Work out the finished part from the listing and answer in its coordinate system (mm). A direction names the side the tool comes from. Give positions to 0.01 mm unless a question says otherwise; leave off trailing zeros. Order: outer loops, then holes, each group sorted by start corner. A loop starts at its lowest first (then second) coordinate and runs counter-clockwise, first axis right, second up.
```python
from build123d import *

# Parameters (mm, degrees)
CROQUIS1_R              = 4
CROQUIS1_R_2            = 3
SALIENTE_EXTRUIR1_DEPTH = 5.5
CROQUIS2_R              = 5.35
CROQUIS2_R_2            = 3
SALIENTE_EXTRUIR2_DEPTH = 2.5
REDONDEO1_R             = 1
CROQUIS3_R              = 4
SALIENTE_EXTRUIR3_DEPTH = 7
CROQUIS4_W              = 2.8
CROQUIS4_H              = 0.7
CROQUIS4_W_2            = 0.7
CROQUIS4_H_2            = 2.8
SALIENTE_EXTRUIR4_DEPTH = 5.3
CROQUIS5_R              = 4
SALIENTE_EXTRUIR5_DEPTH = 2


with BuildPart() as part:
    # Croquis1 → Saliente-Extruir1 (new body)
    with BuildSketch(Plane.XY):
        Circle(CROQUIS1_R)
        Circle(CROQUIS1_R_2, mode=Mode.SUBTRACT)
    extrude(amount=-SALIENTE_EXTRUIR1_DEPTH)

    # Croquis2 → Saliente-Extruir2 (add)
    with BuildSketch(Plane(origin=(0, 0, -5.5), x_dir=(-1, 0, 0), z_dir=(0, 0, -1))):
        Circle(CROQUIS2_R)
        with Locations(Location((0, 0, 0), (0, 0, 180))):
            Circle(CROQUIS2_R_2, mode=Mode.SUBTRACT)
    extrude(amount=SALIENTE_EXTRUIR2_DEPTH)

    # Redondeo1
    redondeo1_edges = [part.edges().sort_by_distance(p)[0] for p in [
        (5.35, 0, -8),
    ]]
    fillet(redondeo1_edges, radius=REDONDEO1_R)

    # Croquis3 → Saliente-Extruir3 (add)
    with BuildSketch(Plane(origin=(0, 0, -8), x_dir=(-1, 0, 0), z_dir=(0, 0, -1))):
        with Locations(Location((0, 0, 0), (0, 0, 180))):
            Circle(CROQUIS3_R)
    extrude(amount=SALIENTE_EXTRUIR3_DEPTH)

    # Croquis4 → Saliente-Extruir4 (add)
    with BuildSketch(Plane(origin=(0, 0, -15), x_dir=(-1, 0, 0), z_dir=(0, 0, -1))):
        with Locations((0, 3.396998799)):
            Rectangle(CROQUIS4_W, CROQUIS4_H)
        with Locations((-3.396998799, 0)):
            Rectangle(CROQUIS4_W_2, CROQUIS4_H_2)
        with Locations((3.396998799, 0)):
            Rectangle(CROQUIS4_W_2, CROQUIS4_H_2)
    extrude(amount=SALIENTE_EXTRUIR4_DEPTH)

    # Croquis5 → Saliente-Extruir5 (add)
    with BuildSketch(Plane.XY):
        Polygon((5.484827557, 0), (2.742413779, 4.75), (-2.742413779, 4.75), (-5.484827557, 0), (-2.742413779, -4.75), (2.742413779, -4.75), align=None)
        Circle(CROQUIS5_R, mode=Mode.SUBTRACT)
    extrude(amount=-SALIENTE_EXTRUIR5_DEPTH)


solid = part.part
```
1. The part is cut by section C-C (z = -13.5). Write down the section's boundary in (x, y), then the cut area to 3 significant figures.
Findings below:
outline: circle Ø8 at (0, 0)
area: 50.3 mm2
2. Straight lines are drawn through the part: probe 1 along Y at (x, z) = (0, -6.65); probe 2 along Z at (x, y) = (0.5, -4); probe 3 along Y at (x, z) = (0, -2.5). For each, find the intervals that lie inside material, in ascending order.
Findings below:
probe 1: y = -5.35 to -3, 3 to 5.35
probe 2: z = -8 to -5.5, -2 to 0
probe 3: y = -4 to -3, 3 to 4
3. The part is cut by section A-A (z = -17). Write down the section's boundary in (x, y).
Findings below:
outline: (-3.75, -1.4) - (-3.05, -1.4) - (-3.05, 1.4) - (-3.75, 1.4) - close; (-1.4, 3.05) - (1.4, 3.05) - (1.4, 3.75) - (-1.4, 3.75) - close; (3.05, -1.4) - (3.75, -1.4) - (3.75, 1.4) - (3.05, 1.4) - close
4. The mould has two halves that part along X. Classify faces 1 (the face through (0, -4.75, -1)), 2 (the face through (1.16, -5.223, -6.24)), 3 (the face through (0, 0, -15)), 4 (the face through (0, 0, -8)): pulls with the +X half, pulls with the -X half, needs draft (parallel to the pull), parting line crosses it, or undercut.
Findings below:
face 1: needs draft
face 2: parting line crosses it
face 3: undercut
face 4: undercut
5. The part is cut by section B-B (x = 0). Write down the section's boundary in (y, z).
Findings below:
outline: (-5.35, -7) arc R1 ccw to (-4.35, -8) - (-4, -8) - (-4, -15) - (3.05, -15) - (3.05, -20.3) - (3.75, -20.3) - (3.75, -15) - (4, -15) - (4, -8) - (4.35, -8) arc R1 ccw to (5.35, -7) - (5.35, -5.5) - (4, -5.5) - (4, -2) - (4.75, -2) - (4.75, 0) - (3, 0) - (3, -8) - (-3, -8) - (-3, 0) - (-4.75, 0) - (-4.75, -2) - (-4, -2) - (-4, -5.5) - (-5.35, -5.5) - close
6. Which of the six approach directions +Z, -Z, +X, -X, +Y, -Y give full straight-line access (tool end or side, diameter ignored) to faces 5 (the face through (4.04, -1.03, -2)), 6 (the face through (-0.867, 3.905, -11.451)), 7 (the face through (4.1, -2.4, -1)), 8 (the face through (3.747, 0, -18))?
Findings below:
face 5: none
face 6: -Z
face 7: +Z, +X, -Y
face 8: -Z, +X, +Y, -Y
7. Given P1, Ø4, axis at y = 2, z = -6, coming from the +X side; P2, Ø1.5, axis at x = -2, z = -7.5, coming from the +Y side; P3, Ø3.5, axis at x = 0, y = 0, coming from the +Z side, each flat-ended and moving along its own axis, determine where each tip first touches the part or whether it passes through.
Findings below:
P1: stops at x = 5.35
P2: stops at y = 5.17
P3: stops at z = -8
8. The part is cut by section D-D (z = -6.5). Write down the section's boundary in (x, y), then the cut area to 3 significant figures.
Findings below:
outline: circle Ø10.7 at (0, 0); hole circle Ø6 at (0, 0)
area: 61.6 mm2
